from build123d import *

# Parameters (mm, degrees)
F0_R      = 72.672804
F1_DEPTH  = 25.4
F2_R      = 20.344191
F3_DEPTH  = 508
F3_FACE_R = 20.344191
F4_DEPTH  = 25.4


with BuildPart() as f1:
    # F0 (on Front) → F1 (new body)
    with BuildSketch(Plane.XZ):
        Circle(F0_R)
    extrude(amount=F1_DEPTH)

    # F2 (on Front) → F3 (join)
    with BuildSketch(Plane.XZ):
        Circle(F2_R)
    extrude(amount=-F3_DEPTH)

    # F3_face (on face) → F4 (join)
    with BuildSketch(Plane(origin=(0, 508, 0), x_dir=(1, 0, 0), z_dir=(0, 1, 0))):
        Circle(F3_FACE_R)
    extrude(amount=F4_DEPTH)


solid = f1.part
Read the model definition and answer for the solid it produces. Units are mm, in the model's axes. A direction names the side the tool comes from. Give positions to 0.01 mm unless a question says otherwise; leave off trailing zeros. Write each loop counter-clockwise with the first axis right and the second up, starting at its lowest first coordinate (ties: lowest second). Pieces come first, ordered by that corner, then holes. Notation, with made-up numbers: (-20.75, -13.75) - (38.25, -13.75) arc R20 ccw to (38.25, 1.25) - close; hole circle Ø9 at (-11.5, 51). An arc over 180 degrees is marked (long way). Return JSON: item names as keys, results as strings.
Q1. Consider line 1 along Y through (x, z) = (53, -11); line 2 along X through (y, z) = (-2, -2.5); line 3 along Z through (x, y) = (9, 291). Determine where each line is inside the solid, lowest interval first. Write a range as [from, to].
Reply:
{"line 1": "[-25.4, 0]", "line 2": "[-72.63, 72.63]", "line 3": "[-18.25, 18.25]"}
Q2. Given P1, Ø5, axis at x = 42.5, z = 28.5, coming from the +Y side; P2, Ø10, axis at y = 150, z = -14, coming from the +X side; P3, Ø8, axis at x = 15, y = 137, coming from the +Z side, each flat-ended and moving along its own axis, determine where each tip first touches the part or whether it passes through.
Reply:
{"P1": "y = 0", "P2": "x = 18.25", "P3": "z = 17.11"}
Q3. For faces 1 (the face through (15, 0, -15)), 2 (the face through (0, 533.4, 0)), determine the directions among +Z, -Z, +X, -X, +Y, -Y from which every point of the face is accessible in a straight line to the end or side of a thin tool.
Reply:
{"face 1": "+Y", "face 2": "+Z, -Z, +X, -X, +Y"}
Q4. A cutting plane is placed at B-B, the plane z = 0. Determine the outline of the cut face in (x, y), and give its area (3 significant figures).
Reply:
{"outline": "(-72.67, -25.4) - (72.67, -25.4) - (72.67, 0) - (20.34, 0) - (20.34, 533.4) - (-20.34, 533.4) - (-20.34, 0) - (-72.67, 0) - close", "area": "25,400 mm²"}
Q5. A cutting plane is placed at D-D, the plane z = 55.5. Determine the outline of the cut face in (x, y), and give its area (3 significant figures).
Reply:
{"outline": "(-46.92, -25.4) - (46.92, -25.4) - (46.92, 0) - (-46.92, 0) - close", "area": "2,380 mm²"}
Q6. A cutting plane is placed at C-C, the plane y = 349.5. Determine the outline of the cut face in (x, z), and give its area (3 significant figures).
Reply:
{"outline": "circle Ø40.69 at (0, 0)", "area": "1,300 mm²"}
Q7. A cutting plane is placed at A-A, the plane x = 0. Determine the outline of the cut face in (y, z), and give its area (3 significant figures).
Reply:
{"outline": "(-25.4, -72.67) - (0, -72.67) - (0, -20.34) - (533.4, -20.34) - (533.4, 20.34) - (0, 20.34) - (0, 72.67) - (-25.4, 72.67) - close", "area": "25,400 mm²"}
